Read the model definition and answer for the solid it produces. Units are mm, in the model's axes. A direction names the side the tool comes from. Coordinates: 2 decimals unless noted, no trailing zeros. Write each loop counter-clockwise with the first axis right and the second up, starting at its lowest first coordinate (ties: lowest second). Pieces come first, ordered by that corner, then holes.
Item 1: Determine the mould class of faces 1 (the face through (-2, 35, 7)), 2 (the face through (-8, 25, 7)), 3 (the face through (-15.432, 11.946, 12.465)), 4 (the face through (-1, -2, 5)) for opening direction Y: released by +Y, released by -Y, zero draft, split by the parting line, or undercut.
Item 2: Section D-D (x = -16) is taken. Give the vertices of the cut face in (y, z), then the cut area to 3 significant figures.
Item 3: Straight lines are drawn through the part: probe 1 along Z at (x, y) = (5.5, -9); probe 2 along Z at (x, y) = (-15.5, 10); probe 3 along Y at (x, z) = (-10, 3). For each, find the intervals that lie inside material, in ascending order.
Item 4: Section C-C (z = 3) is taken. Give the vertices of the cut face in (x, y).
Item 5: Section A-A (x = -5) is taken. Give the vertices of the cut face in (y, z).
Item 6: Each of these flat-tipped pins is pushed along its axis until it touches: P1, Ø8, axis at x = -17, z = 6.5, coming from the +Y side; P2, Ø4, axis at y = 21.5, z = 7.5, coming from the -X side; P3, Ø1.5, axis at x = -19, z = 12.5, coming from the +Y side. Where does it stop, or does it pass through?
Item 7: A tool of negligible diameter and unlimited length cuts with its end or side. For faces 5 (the face through (-7, 7, 4)), 6 (the face through (-5.74, 0.1, 2.54)), 7 (the face through (-9.261, 5.775, 7.535)), 8 (the face through (-14, 9, 10)), from which of +Z, -Z, +X, -X, +Y, -Y can it reach the whole face along a straight path? Write none if from no direction.
Item 8: Section B-B (y = 1.5) is taken. Give the vertices of the cut face in (x, z).
from build123d import *

# Parameters (mm, degrees)
EXTRUDE_1_DEPTH     = 10
SKETCH_2_R          = 1.5
CUT_EXTRUDE_1_DEPTH = 10
SKETCH_3_R          = 1.5
CUT_EXTRUDE_4_DEPTH = 5
SKETCH_4_W          = 5
SKETCH_4_H          = 5
CUT_EXTRUDE_5_DEPTH = 5
EXTRUDE_2_DEPTH     = 5


with BuildPart() as part:
    # 草图1 → 凸台-拉伸1 (new body)
    with BuildSketch(Plane.XY):
        Polygon((-23.571067812, 16.5), (5, -12.071067812), (8.535533906, -8.535533906), (6.051882873, -6.051882873), (0, 0), (-16.5, 16.5), (0, 33), (-3.535533906, 36.535533906), align=None)
    extrude(amount=EXTRUDE_1_DEPTH)

    # 草图2 → 切除-拉伸1 (cut)
    with BuildSketch(Plane.XY.offset(10)):
        with Locations((-4.550561614, 1.015027708)):
            Circle(SKETCH_2_R)
    extrude(amount=-CUT_EXTRUDE_1_DEPTH, mode=Mode.SUBTRACT)

    # 草图3 → 切除-拉伸4 (cut)
    with BuildSketch(Plane.XY.offset(10)):
        Polygon((-1.596461706, 6.368004388), (-3.982233047, 3.982233047), (8.535533906, -8.535533906), (5, -12.071067812), (-7.517766953, 0.446699141), (-9.33715939, -1.372693296), (6.144235978, -17.323833909), (15.036478659, -7.320060893), align=None)
        Polygon((8.535533906, -8.535533906), (-3.982233047, 3.982233047), (-4.279030417, 3.685435677), (-7.517766953, 0.446699141), (5, -12.071067812), align=None)
        with Locations((-4.550561614, 1.015027708)):
            Circle(SKETCH_3_R, mode=Mode.SUBTRACT)
    extrude(amount=-CUT_EXTRUDE_4_DEPTH, mode=Mode.SUBTRACT)

    # 草图4 → 切除-拉伸5 (cut)
    with BuildSketch(Plane(origin=(-3.982233047, 3.982233047, 0), x_dir=(0, 0, -1), z_dir=(0.707106781, -0.707106781, 0))):
        with Locations((-7.5, -2.5)):
            Rectangle(SKETCH_4_W, SKETCH_4_H)
    extrude(amount=-CUT_EXTRUDE_5_DEPTH, mode=Mode.SUBTRACT)

    # 草图5 → 凸台-拉伸2 (add)
    with BuildSketch(Plane.XY.offset(10)):
        Polygon((-7.517766953, 7.517766953), (-23.571067812, 16.5), (-3.535533906, 36.535533906), (0, 33), (-16.5, 16.5), align=None)
    extrude(amount=EXTRUDE_2_DEPTH)


solid = part.part
Established:
1. face 1: released by +Y
1. face 2: undercut
1. face 3: released by -Y
1. face 4: zero draft
2. outline: (8.93, 0) - (16, 0) - (16, 15) - (12.26, 15) - (12.26, 10) - (8.93, 10) - close; (17, 0) - (24.07, 0) - (24.07, 15) - (17, 15) - close
2. area: 195 mm2
3. probe 1: z = 0 to 5
3. probe 2: z = 0 to 10
3. probe 3: y = 2.93 to 10, 23 to 30.07
4. outline: (-23.57, 16.5) - (5, -12.07) - (8.54, -8.54) - (-16.5, 16.5) - (0, 33) - (-3.54, 36.54) - close; hole circle Ø3 at (-4.55, 1.02)
5. outline: (-2.07, 0) - (-0.42, 0) - (-0.42, 5) - (-2.07, 5) - close; (2.45, 0) - (5, 0) - (5, 5) - (2.45, 5) - close; (28, 0) - (35.07, 0) - (35.07, 15) - (28, 15) - close
6. P1: stops at y = 27.07
6. P2: stops at x = -20.57
6. P3: stops at y = 21.82
7. face 5: +Z, -Z, +X
7. face 6: +Z, -Z
7. face 7: +Z, +X, -Y
7. face 8: +Z, -X, -Y
8. outline: (-8.57, 0) - (-5.97, 0) - (-5.97, 5) - (-8.57, 5) - close; (-3.13, 0) - (-1.5, 0) - (-1.5, 5) - (-3.13, 5) - close
